Here's the drawing with two shaded views (mm, measured from the low corner). I have some questions. Round coordinates to 2 decimals unless told otherwise and drop trailing zeros. Loops run counter-clockwise (first coordinate to the right, second up) from the corner with the lowest first, then second, coordinate; pieces in that order, holes last. Notation, with made-up numbers: (42, -21) - (81, -21) arc R13 ccw to (81, -14) - close; hole circle Ø6 at (3.25, 85). An arc over 180 degrees is marked (long way). Use one line per item in the form item = value.
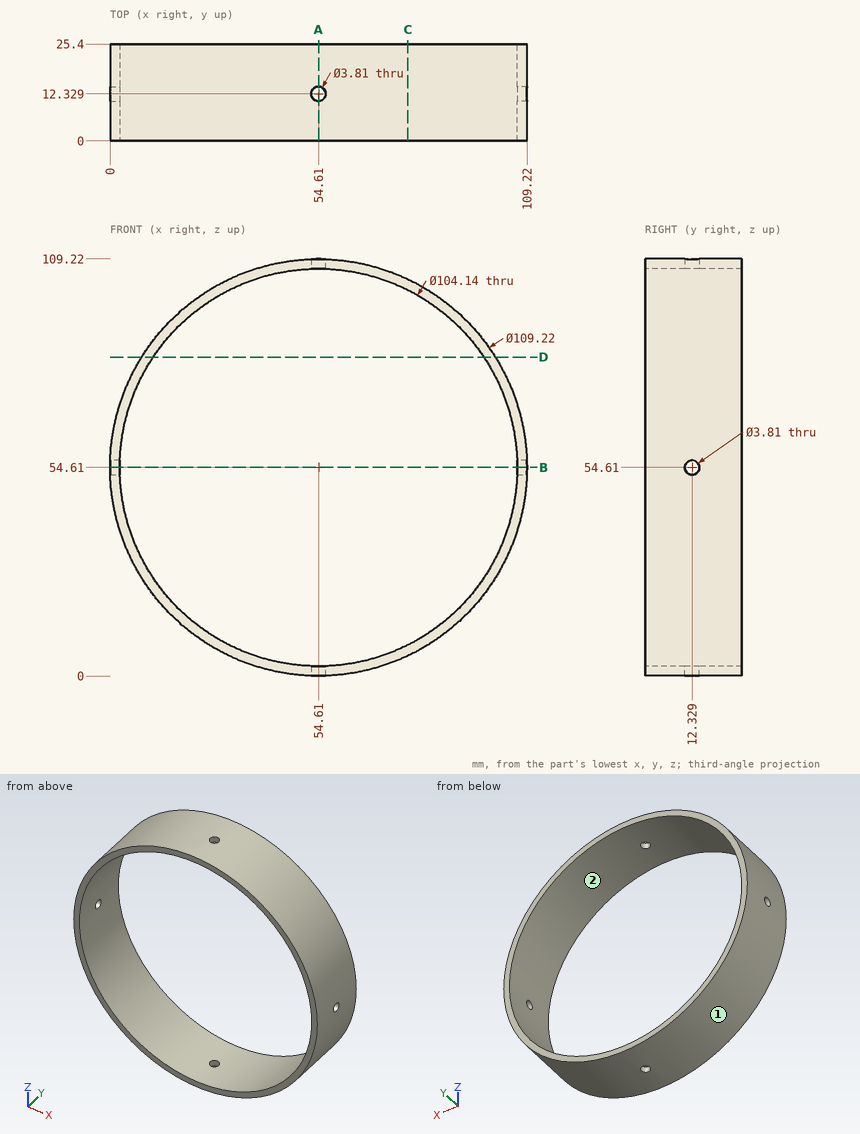
1. Please list where these lines run through material, in increasing order: line 1 along Y through (x, z) = (54.61, 0.75); line 2 along Z through (x, y) = (88, 12) (3 decimals); line 3 along Z through (x, y) = (54, 24).
Solution:
line_1 = 0 to 10.42, 14.23 to 25.4
line_2 = 11.397 to 14.655, 94.565 to 97.823
line_3 = 0 to 2.54, 106.68 to 109.22
2. If we section it at C-C, the plane x = 78: Write out the boundary of the cut face in (y, z), plus the area to 3 significant figures.
Solution:
outline = (0, 5.26) - (25.4, 5.26) - (25.4, 8.09) - (0, 8.09) - close; (0, 101.13) - (25.4, 101.13) - (25.4, 103.96) - (0, 103.96) - close
area = 144 mm^2
3. For P1, Ø2, axis at y = 16.5, z = 12, coming from the +X side; P2, Ø3, axis at y = 12.33, z = 54.61, coming from the +X side; P3, Ø12, axis at y = 16.5, z = 35, coming from the +X side; P4, Ø2, axis at y = 21, z = 35.5, coming from the +X side, each with a flat end and sliding along its axis, tell me the tip position at first contact or that it passes through.
Solution:
P1 = 89.98
P2 = through
P3 = 107.5
P4 = 106.13
4. We'd pull the mould along X, two halves only. Please class the marked faces 1 and 2: +X half, -X half, draft (parallel to the pull), parting line (faces both ways), or undercut.
Solution:
face_1 = parting line
face_2 = undercut
5. If we section it at A-A, the plane x = 54.61: Write out the boundary of the cut face in (y, z), plus the area to 3 significant figures.
Solution:
outline = (0, 0) - (10.42, 0) - (10.42, 2.54) - (0, 2.54) - close; (0, 106.68) - (10.42, 106.68) - (10.42, 109.22) - (0, 109.22) - close; (14.23, 0) - (25.4, 0) - (25.4, 2.54) - (14.23, 2.54) - close; (14.23, 106.68) - (25.4, 106.68) - (25.4, 109.22) - (14.23, 109.22) - close
area = 110 mm^2
6. If we section it at B-B, the plane z = 54.61: Write out the boundary of the cut face in (x, y).
Solution:
outline = (0, 0) - (2.54, 0) - (2.54, 10.42) - (0, 10.42) - close; (0, 14.23) - (2.54, 14.23) - (2.54, 25.4) - (0, 25.4) - close; (106.68, 0) - (109.22, 0) - (109.22, 10.42) - (106.68, 10.42) - close; (106.68, 14.23) - (109.22, 14.23) - (109.22, 25.4) - (106.68, 25.4) - close
7. If we section it at D-D, the plane z = 83.5: Write out the boundary of the cut face in (x, y).
Solution:
outline = (8.27, 0) - (11.29, 0) - (11.29, 25.4) - (8.27, 25.4) - close; (97.93, 0) - (100.95, 0) - (100.95, 25.4) - (97.93, 25.4) - close
